from build123d import *

# Parameters (mm, degrees)
PAD_DEPTH    = 3
SKETCH001_R  = 1.5
PAD001_DEPTH = 7.25
SKETCH002_R  = 2.1
POCKET_DEPTH = 2


with BuildPart() as part:
    # Sketch → Pad (new body)
    with BuildSketch(Plane.XY):
        Polygon((-7.75, 33), (-7.75, -33), (15.75, -33), (15.75, -11.5), (7.75, -11.5), (7.75, 33), (5, 33), (5, 43), (-5, 43), (-5, 33), align=None)
    extrude(amount=PAD_DEPTH)

    # Sketch001 → Pad001 (join, symmetric)
    with BuildSketch(Plane.YZ):
        with Locations((40, 1.5)):
            Circle(SKETCH001_R)
    extrude(amount=PAD001_DEPTH, both=True)

    # Sketch002 (on Face5 of Pad001) → Pocket (cut)
    with BuildSketch(Plane.XY.offset(3)):
        with Locations((4, -23)):
            Circle(SKETCH002_R)
    extrude(amount=-POCKET_DEPTH, mode=Mode.SUBTRACT)


solid = part.part
Design review of the part built by this model. Coordinates are the model's own, in mm. A direction names the side the tool comes from. Coordinates: 2 decimals unless noted, no trailing zeros. Order: outer loops, then holes, each group sorted by start corner. A loop starts at its lowest first (then second) coordinate and runs counter-clockwise, first axis right, second up.
Item 1: For faces 5 (the flat face through (6, 33, 1)), 6 (the flat face through (4, -23, 1)), 7 (the flat face through (12, -11.5, 1)), list the 3-axis set-ups (+Z, -Z, +X, -X, +Y, -Y) from which the entire face can be reached by the end or side of a thin tool; tool diameter is ignored.
Item 2: For pin 1 Ø1.5 at (y, z) = (36.5, 1) entering from -X; pin 2 Ø1.5 at (y, z) = (39.5, 1) entering from +X; pin 3 Ø0.8 at (x, z) = (7, 1.5) entering from +Y, all flat-tipped, find the tip position at first contact; note any pin that passes through.
Item 3: The part is to be moulded in two halves that separate along Y. For faces 1 (the flat face through (5, 36, 1)), 2 (the flat face through (4, -33, 1)), 3 (the flat face through (-5, 36, 1)), 4 (the flat face through (1, -3, 3)), say which applies: pulls with the +Y half, pulls with the -Y half, needs draft (parallel to the pull), parting line crosses it, or undercut.
Item 4: Take a section at B-B, the plane y = -23. Write out the cut boundary in (x, z).
Item 5: For line 1 (Y direction, x = -5.25, z = 1.7); line 2 (Y direction, x = 4, z = 2.35); line 3 (X direction, y = 15.5, z = 1.7), list the stretches that pass through material, from the lowest coordinate up.
Item 6: Take a section at D-D, the plane x = 13. Write out the cut boundary in (y, z).
Item 7: Take a section at A-A, the plane z = 1.5. Write out the cut boundary in (x, y).
Item 8: Take a section at C-C, the plane x = 4. Write out the cut boundary in (y, z), then the cut area to 3 significant figures.
The answers:
1. face 5: +Z, -Z, +X
1. face 6: +Z
1. face 7: +Z, -Z, +X, +Y
2. pin 1: stops at x = -5
2. pin 2: stops at x = 7.25
2. pin 3: stops at y = 41.5
3. face 1: undercut
3. face 2: pulls with the -Y half
3. face 3: undercut
3. face 4: needs draft
4. outline: (-7.75, 0) - (15.75, 0) - (15.75, 3) - (6.1, 3) - (6.1, 1) - (1.9, 1) - (1.9, 3) - (-7.75, 3) - close
5. line 1: y = -33 to 33, 38.51 to 41.49
5. line 2: y = -33 to -25.1, -20.9 to 43
5. line 3: x = -7.75 to 7.75
6. outline: (-33, 0) - (-11.5, 0) - (-11.5, 3) - (-33, 3) - close
7. outline: (-7.75, -33) - (15.75, -33) - (15.75, -11.5) - (7.75, -11.5) - (7.75, 33) - (5, 33) - (5, 38.5) - (7.25, 38.5) - (7.25, 41.5) - (5, 41.5) - (5, 43) - (-5, 43) - (-5, 41.5) - (-7.25, 41.5) - (-7.25, 38.5) - (-5, 38.5) - (-5, 33) - (-7.75, 33) - close; hole circle Ø4.2 at (4, -23)
8. outline: (-33, 0) - (43, 0) - (43, 3) - (-20.9, 3) - (-20.9, 1) - (-25.1, 1) - (-25.1, 3) - (-33, 3) - close
8. area: 220 mm2
